```python
from build123d import *

# Parameters (mm, degrees)
F1_DEPTH    = 3
F3_DEPTH    = 5
F4_T1_DEPTH = 20
F4_T3_DEPTH = 18.7590602534
F4_T5_DEPTH = 18.4414894703
F5_T1_DEPTH = 28.8976125792
F5_T3_DEPTH = 28.7


# Not quite as in the source:
# - a fillet or chamfer that OpenCascade refuses, or shapes differently, is made with other operations: its cross-section is extruded or revolved along the edge and cut away or added


with BuildPart() as f1:
    # F0 (on Top) → F1 (new body)
    with BuildSketch(Plane.XY):
        with BuildLine():
            ThreePointArc((-2.8925442436, -3.447199994), (0, 4.5), (2.8925442436, -3.447199994))
            Line((2.8925442436, -3.447199994), (3.8567256581, -4.5962666587))
            ThreePointArc((3.8567256581, -4.5962666587), (5.9714768944, 0.5843489538), (2.8925442436, 5.2567278605))
            ThreePointArc((2.8925442436, 5.2567278605), (2.2135929139, 5.5767379723), (1.5, 5.8094750193))
            Line((1.5, 5.8094750193), (1.5, 8.2567278605))
            Line((1.5, 8.2567278605), (-1.5, 8.2567278605))
            Line((-1.5, 8.2567278605), (-1.5, 5.8094750193))
            ThreePointArc((-1.5, 5.8094750193), (-5.8517939481, 1.3253330104), (-3.8567256581, -4.5962666587))
            Line((-3.8567256581, -4.5962666587), (-2.8925442436, -3.447199994))
        make_face()
    extrude(amount=F1_DEPTH)

    # F2 (on face) → F3 (join)
    with BuildSketch(Plane(origin=(0, 8.2567278605, 0), x_dir=(-1, 0, 0), z_dir=(0, 1, 0))):
        Polygon((-15, 0), (-5, 0), (-5, -28.8976125792), (-8, -28.8976125792), (-8, -31.8976125792), (8, -31.8976125792), (8, -28.8976125792), (5, -28.8976125792), (5, 0), (15, 0), (15, 3), (15, 8), (15, 11.5052), (9.8263609009, 11.5052), (9.8263609009, 8), (11.4948, 8), (11.4948, 3), (0, 3), (-11.4948, 3), (-11.4948, 8), (-9.6895930523, 8), (-9.6895930523, 11.5052), (-13.1947930523, 11.5052), (-15, 11.5052), (-15, 8), (-15, 3), align=None)
    extrude(amount=F3_DEPTH)

    # F4: fillet of radius 3 on 4 edges, made by hand

    # F4_s2 → F4_t1 (cut)
    with BuildSketch(Plane.XZ.offset(-20.7567278605)):
        with BuildLine():
            ThreePointArc((12.6895930523, 11.5052), (10.5682727087, 10.6265203436), (9.6895930523, 8.5052))
            Line((9.6895930523, 8.5052), (9.6895930523, 11.5052))
            Line((9.6895930523, 11.5052), (12.6895930523, 11.5052))
        make_face()
        with BuildLine():
            ThreePointArc((-9.8263609009, 8.5052), (-10.7050405574, 10.6265203436), (-12.8263609009, 11.5052))
            Line((-12.8263609009, 11.5052), (-9.8263609009, 11.5052))
            Line((-9.8263609009, 11.5052), (-9.8263609009, 8.5052))
        make_face()
    extrude(amount=F4_T1_DEPTH, mode=Mode.SUBTRACT)

    # F4_s4 → F4_t3 (cut)
    with BuildSketch(Plane.XZ.offset(-20.1362579871)):
        with BuildLine():
            ThreePointArc((9.6895930523, 10.7518120507), (10.1811693284, 9.1062694588), (11.4948, 8))
            Line((11.4948, 8), (9.6895930523, 8))
            Line((9.6895930523, 8), (9.6895930523, 10.7518120507))
        make_face()
    extrude(amount=F4_T3_DEPTH, mode=Mode.SUBTRACT)

    # F4_s6 → F4_t5 (cut)
    with BuildSketch(Plane.XZ.offset(-19.9774725956)):
        with BuildLine():
            ThreePointArc((-11.4948, 8), (-10.2773726013, 9.1063185489), (-9.8263609009, 10.6882978941))
            Line((-9.8263609009, 10.6882978941), (-9.8263609009, 8))
            Line((-9.8263609009, 8), (-11.4948, 8))
        make_face()
    extrude(amount=F4_T5_DEPTH, mode=Mode.SUBTRACT)

    # F5: fillet of radius 2.54 on 6 edges, made by hand

    # F5_s2 → F5_t1 (cut)
    with BuildSketch(Plane.XY.offset(-28.8976125792)):
        with BuildLine():
            ThreePointArc((5, 10.7167278605), (4.2560512242, 12.5127790847), (2.46, 13.2567278605))
            Line((2.46, 13.2567278605), (5, 13.2567278605))
            Line((5, 13.2567278605), (5, 10.7167278605))
        make_face()
        with BuildLine():
            ThreePointArc((5, 10.7967278605), (4.2560512242, 9.0006766362), (2.46, 8.2567278605))
            Line((2.46, 8.2567278605), (5, 8.2567278605))
            Line((5, 8.2567278605), (5, 10.7967278605))
        make_face()
        with BuildLine():
            ThreePointArc((-2.46, 8.2567278605), (-4.2560512242, 9.0006766362), (-5, 10.7967278605))
            Line((-5, 10.7967278605), (-5, 8.2567278605))
            Line((-5, 8.2567278605), (-2.46, 8.2567278605))
        make_face()
        with BuildLine():
            ThreePointArc((-2.46, 13.2567278605), (-4.2560512242, 12.5127790847), (-5, 10.7167278605))
            Line((-5, 10.7167278605), (-5, 13.2567278605))
            Line((-5, 13.2567278605), (-2.46, 13.2567278605))
        make_face()
    extrude(amount=F5_T1_DEPTH, mode=Mode.SUBTRACT)

    # F5_s4 → F5_t3 (cut)
    with BuildSketch(Plane.YZ.offset(-14.35)):
        with BuildLine():
            ThreePointArc((8.2567278605, -29.3576125792), (9.0006766362, -31.1536638034), (10.7967278605, -31.8976125792))
            Line((10.7967278605, -31.8976125792), (8.2567278605, -31.8976125792))
            Line((8.2567278605, -31.8976125792), (8.2567278605, -29.3576125792))
        make_face()
        with BuildLine():
            ThreePointArc((13.2567278605, -29.3576125792), (12.5127790847, -31.1536638034), (10.7167278605, -31.8976125792))
            Line((10.7167278605, -31.8976125792), (13.2567278605, -31.8976125792))
            Line((13.2567278605, -31.8976125792), (13.2567278605, -29.3576125792))
        make_face()
    extrude(amount=F5_T3_DEPTH, mode=Mode.SUBTRACT)


solid = f1.part
```
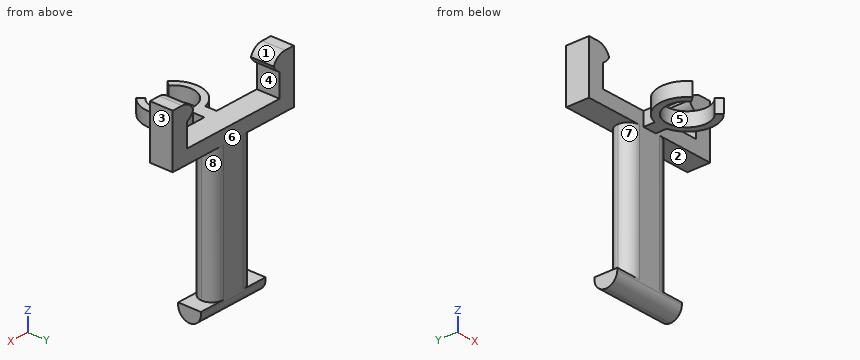
CAD build for the part. Positions are in the model's coordinates, mm. Face numbers are marked on the shaded views. A direction names the side the tool comes from. Round coordinates to 2 decimals unless told otherwise and drop trailing zeros. Loops run counter-clockwise (first coordinate to the right, second up) from the corner with the lowest first, then second, coordinate; pieces in that order, holes last. Notation, with made-up numbers: M 48,70.5 L 101,70.5 A24 cw 101,89.5 Z; hole C 85,77 d7. An arc over 180 degrees is marked long. Use a Markdown table: item, result. Add a question column.
(1) Flat gauge pins, fed straight in: pin 1 (8 mm diameter, centred on x = -4, y = 6.5, fed in from +Z); pin 2 (2.5 mm diameter, centred on y = 6.5, z = 1, fed in from +X); pin 3 (2.5 mm diameter, centred on y = 11, z = -30, fed in from +X); pin 4 (10 mm diameter, centred on y = 9.5, z = -4, fed in from -X). Where does each tip first touch, or does it go through?
(2) Cut at A-A (x = 7.25). Give the cut face in (y, z), and give its area (3 significant figures).
(3) Pull direction X, two halves, no side cores. Call the marked faces 1, 2 and 3: +X half, -X half, draft (parallel to the pull), parting line (faces both ways), or undercut.
(4) Cut at B-B (y = 0). Give the cut face in (x, z), and give its area (3 significant figures).
(5) Drill centre lines: line 1 (X direction, y = 0, z = 1.4); line 2 (Y direction, x = 0, z = 1.15); line 3 (Z direction, x = -0.75, y = 6.5). Where is each one in solid material? Low to high.
(6) Cut at C-C (z = 4). Give the cut face in (x, y).
(7) Cut at D-D (x = 0). Give the cut face in (y, z).
(8) Which spindle directions (+Z, -Z, +X, -X, +Y, -Y) get a long thin tool onto all of the face, cutting with end or side? Do the marked faces 4, 5, 6, 7 and 8. Say none if no direction does.
Geometry says:
| question | item | result |
|---|---|---|
| 1 | pin 1 | stops at z = 3 |
| 1 | pin 2 | stops at x = 2.9 |
| 1 | pin 3 | stops at x = 8 |
| 1 | pin 4 | stops at x = -15 |
| 2 | outline | M 8.26,-29.36 A2.54 ccw 10.76,-31.9 A2.54 ccw 13.26,-29.36 L 13.26,-28.9 L 8.26,-28.9 Z; M 8.26,0 L 13.26,0 L 13.26,3 L 8.26,3 Z |
| 2 | area | 27.2 mm² |
| 3 | face 1 | undercut |
| 3 | face 2 | draft |
| 3 | face 3 | +X half |
| 4 | outline | M -6,0 L -4.5,0 L -4.5,3 L -6,3 Z; M 4.5,0 L 6,0 L 6,3 L 4.5,3 Z |
| 4 | area | 9.00 mm² |
| 5 | line 1 | x = -6 to -4.5, 4.5 to 6 |
| 5 | line 2 | y = 4.5 to 13.26 |
| 5 | line 3 | z = 0 to 3 |
| 6 | outline | M -15,8.26 L -11.49,8.26 L -11.49,13.26 L -15,13.26 Z; M 11.49,8.26 L 15,8.26 L 15,13.26 L 11.49,13.26 Z |
| 7 | outline | M 4.5,0 L 8.26,0 L 8.26,-29.36 A2.54 ccw 10.76,-31.9 A2.54 ccw 13.26,-29.36 L 13.26,3 L 4.5,3 Z |
| 8 | face 4 | +Y, -Y |
| 8 | face 5 | +Z, -Z |
| 8 | face 6 | +Z, -Z, +X, -X, +Y |
| 8 | face 7 | -X, -Y |
| 8 | face 8 | +X, +Y |
